Verification items for this drawing (mm, ordinates from the low corner). A direction names the side the tool comes from. Coordinates: 2 decimals unless noted, no trailing zeros. Order: outer loops, then holes, each group sorted by start corner. A loop starts at its lowest first (then second) coordinate and runs counter-clockwise, first axis right, second up. Notation, with made-up numbers: (36, -32.5) -> (62, -32.5) arc R21 ccw to (62, 0.5) -> close; hole circle Ø7 at (33.5, 71). An arc over 180 degrees is marked (long way). Write each question's results on one line, items separated by ' | '. Start each with the question number.
(1) Draft check along Y on the marked faces 1, 2 and 3. Enter one of: +Y half, -Y half, draft (parallel to the pull), parting line (faces both ways), or undercut.
(2) Set-up check for the marked faces 4 and 5: record each of +Z, -Z, +X, -X, +Y, -Y from which the full face is reachable in a straight line by a thin tool's end or side.
(3) Thickness scan on probe 1 along X at (y, z) = (161.5, 522); probe 2 along Z at (x, y) = (183, 84); probe 3 along Z at (x, y) = (131, 127.5). Record the ranges inside material, lowest first. Write a range as [from, to].
(4) Cross-section at B-B on x = 147.5. Enter the section's corners in (y, z).
(5) Cross-section at C-C on z = 334.5. Enter the section's corners in (x, y), and give its area (3 significant figures).
(6) Go/stop test with a flat-tipped pin: pin 1 (10 mm diameter, centred on x = 77.5, y = 41.5, fed in from -Z). Record where the tip stops, or that it passes through.
(7) Cross-section at D-D on y = 25.4. Enter the section's corners in (x, z), and give its area (3 significant figures).
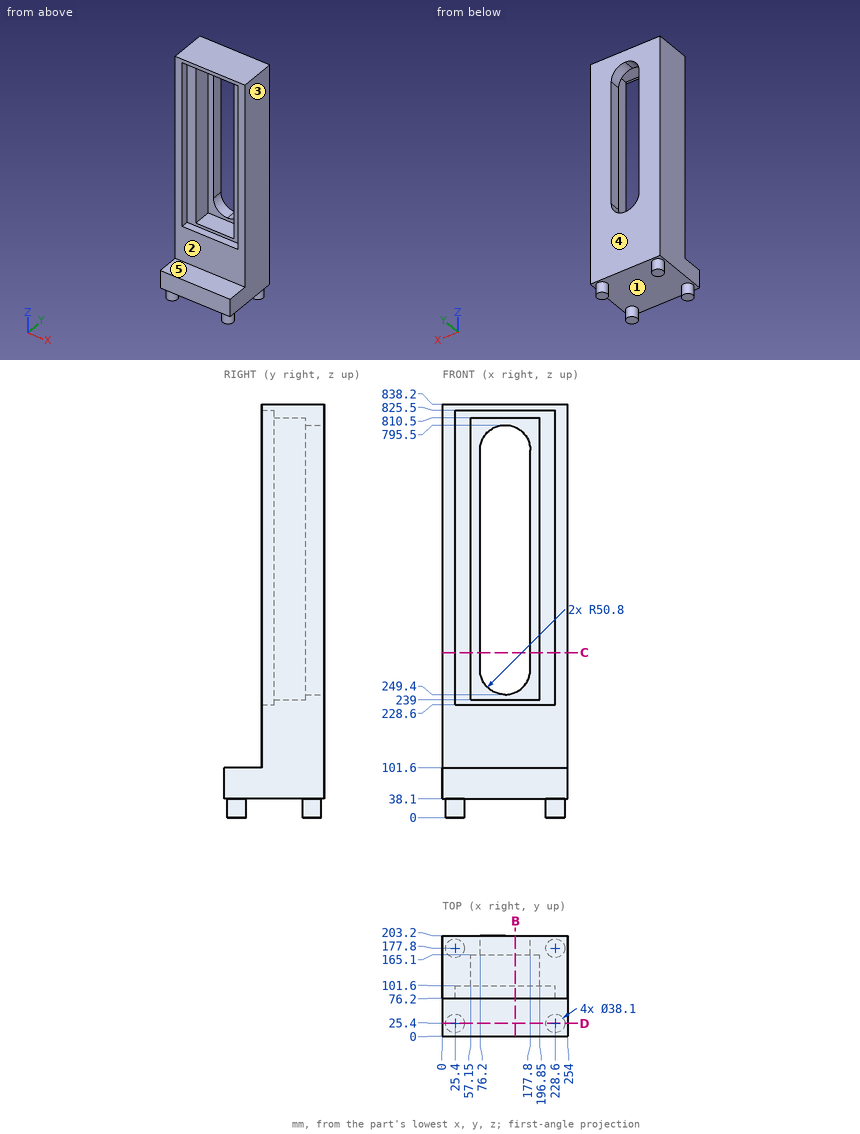
Results are:
1) face 1: undercut | face 2: -Y half | face 3: draft
2) face 4: +Z, -Z, +X, -X, +Y | face 5: +Z, +X, -X, -Y
3) probe 1: x = [0, 57.15], [196.85, 254] | probe 2: z = [38.1, 228.6], [825.5, 838.2] | probe 3: z = [38.1, 239], [810.5, 838.2]
4) outline: (0, 38.1) -> (203.2, 38.1) -> (203.2, 253.72) -> (165.1, 253.72) -> (165.1, 239) -> (101.6, 239) -> (101.6, 228.6) -> (76.2, 228.6) -> (76.2, 101.6) -> (0, 101.6) -> close; (76.2, 825.5) -> (101.6, 825.5) -> (101.6, 810.5) -> (165.1, 810.5) -> (165.1, 791.18) -> (203.2, 791.18) -> (203.2, 838.2) -> (76.2, 838.2) -> close
5) outline: (0, 76.2) -> (25.4, 76.2) -> (25.4, 101.6) -> (57.15, 101.6) -> (57.15, 165.1) -> (76.2, 165.1) -> (76.2, 203.2) -> (0, 203.2) -> close; (177.8, 165.1) -> (196.85, 165.1) -> (196.85, 101.6) -> (228.6, 101.6) -> (228.6, 76.2) -> (254, 76.2) -> (254, 203.2) -> (177.8, 203.2) -> close | area: 14,400 mm2
6) pin 1: stops at z = 38.1
7) outline: (0, 38.1) -> (6.35, 38.1) -> (6.35, 0) -> (44.45, 0) -> (44.45, 38.1) -> (209.55, 38.1) -> (209.55, 0) -> (247.65, 0) -> (247.65, 38.1) -> (254, 38.1) -> (254, 101.6) -> (0, 101.6) -> close | area: 19,000 mm2
